from build123d import *

# Parameters (mm, degrees)
SKETCH1_W           = 7.62
SKETCH1_H           = 20.066
BOSS_EXTRUDE1_DEPTH = 6.35
BOSS_EXTRUDE2_DEPTH = 20.066


with BuildPart() as part:
    # Sketch1 → Boss-Extrude1 (new body)
    with BuildSketch(Plane.XY):
        with Locations((3.81, 10.033)):
            Rectangle(SKETCH1_W, SKETCH1_H)
    extrude(amount=BOSS_EXTRUDE1_DEPTH)

    # Sketch4 → Boss-Extrude2 (add)
    with BuildSketch(Plane.XZ):
        Polygon((0, 6.35), (1.397, 9.525), (6.223, 9.525), (7.62, 6.35), align=None)
    extrude(amount=-BOSS_EXTRUDE2_DEPTH)


solid = part.part
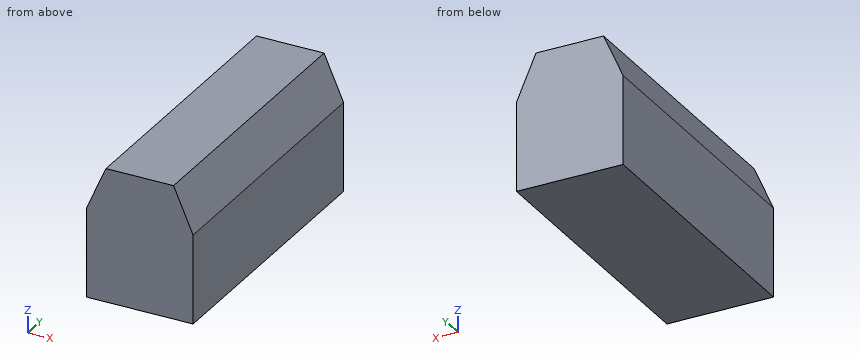
Verification items for the finished model (mm, model axes). Give positions to 0.01 mm unless a question says otherwise; leave off trailing zeros. Write each loop counter-clockwise with the first axis right and the second up, starting at its lowest first coordinate (ties: lowest second). Pieces come first, ordered by that corner, then holes. Notation, with made-up numbers: (21, 45) -> (38, 45) arc R18 ccw to (38, 71) -> close; hole circle Ø11 at (15, -6). An arc over 180 degrees is marked (long way). Use CSV: the item, a comma, the result in double quotes.
(1) Sectioned sample at B-B (z = 8.25). Record the cut outline in (x, y).
Derived:
outline,"(0.84, 0) -> (6.78, 0) -> (6.78, 20.07) -> (0.84, 20.07) -> close"
(2) Material ranges on L1, parallel to X at y = 1.5, z = 9.25; L2, parallel to X at y = 8, z = 7; L3, parallel to Z at x = 0.5, y = 7.75, recorded low to high.
Derived:
L1,"x = 1.28 to 6.34"
L2,"x = 0.29 to 7.33"
L3,"z = 0 to 7.49"
(3) Sectioned sample at A-A (y = 7.25). Record the cut outline in (x, z) (3 decimals).
Derived:
outline,"(0, 0) -> (7.62, 0) -> (7.62, 6.35) -> (6.223, 9.525) -> (1.397, 9.525) -> (0, 6.35) -> close"
(4) Go/stop test with a flat-tipped pin: pin 1 (1 mm diameter, centred on y = 10.5, z = 7.5, fed in from -X). Record where the tip stops, or that it passes through.
Derived:
pin 1,"stops at x = 0.29"
